```python
from build123d import *

# Parameters (mm, degrees)
SKETCH1_W             = 12
SKETCH1_H             = 12
SKETCH1_R             = 1.65
BOSS_EXTRUDE1_DEPTH   = 7
BOSS_EXTRUDE1_2_DEPTH = 7
BOSS_EXTRUDE1_3_DEPTH = 7
BOSS_EXTRUDE1_4_DEPTH = 7
CUT_EXTRUDE1_START    = -2.25
CUT_EXTRUDE1_DEPTH    = 2.5
SKETCH3_W             = 22
SKETCH3_H             = 12
BOSS_EXTRUDE2_DEPTH   = 7
SKETCH4_W             = 10
SKETCH4_H             = 12
SKETCH4_R             = 1.65
SKETCH4_W_2           = 12
BOSS_EXTRUDE3_DEPTH   = 7
CUT_EXTRUDE2_START    = -2.25
CUT_EXTRUDE2_DEPTH    = 2.5
SKETCH6_W             = 10
SKETCH6_H             = 12
SKETCH6_R             = 1.65
SKETCH6_W_2           = 12
BOSS_EXTRUDE4_DEPTH   = 5


with BuildPart() as part:
    # Sketch1 → Boss-Extrude1 (new body)
    with BuildSketch(Plane(origin=(0, 0, 0), x_dir=(1, 0, 0), z_dir=(0, 1, 0))):
        with Locations((1, 38)):
            Rectangle(SKETCH1_W, SKETCH1_H)
        with Locations((1, 38)):
            Circle(SKETCH1_R, mode=Mode.SUBTRACT)
    extrude(amount=BOSS_EXTRUDE1_DEPTH)


with BuildPart() as body_2:
    # Sketch1 → Boss-Extrude1 2 (new body)
    with BuildSketch(Plane(origin=(0, 0, 0), x_dir=(1, 0, 0), z_dir=(0, 1, 0))):
        with Locations((6, -6)):
            Rectangle(SKETCH1_W, SKETCH1_H)
        with Locations((6, -6)):
            Circle(SKETCH1_R, mode=Mode.SUBTRACT)
    extrude(amount=BOSS_EXTRUDE1_2_DEPTH)


with BuildPart() as body_3:
    # Sketch1 → Boss-Extrude1 3 (new body)
    with BuildSketch(Plane(origin=(0, 0, 0), x_dir=(1, 0, 0), z_dir=(0, 1, 0))):
        with Locations((-10, 18)):
            Rectangle(SKETCH1_W, SKETCH1_H)
        with Locations((-10, 18)):
            Circle(SKETCH1_R, mode=Mode.SUBTRACT)
    extrude(amount=BOSS_EXTRUDE1_3_DEPTH)


with BuildPart() as body_4:
    # Sketch1 → Boss-Extrude1 4 (new body)
    with BuildSketch(Plane(origin=(0, 0, 0), x_dir=(1, 0, 0), z_dir=(0, 1, 0))):
        with Locations((24, 18)):
            Rectangle(SKETCH1_W, SKETCH1_H)
        with Locations((24, 18)):
            Circle(SKETCH1_R, mode=Mode.SUBTRACT)
    extrude(amount=BOSS_EXTRUDE1_4_DEPTH)


with BuildPart() as cut_extrude1_tool:
    # Sketch2 → Cut-Extrude1 (new body)
    with BuildSketch(Plane(origin=(0, 7, 0), x_dir=(1, 0, 0), z_dir=(0, 1, 0)).offset(CUT_EXTRUDE1_START)):
        Polygon((9.233161507, -6), (7.616580754, -3.2), (4.383419246, -3.2), (2.766838493, -6), (4.383419246, -8.8), (7.616580754, -8.8), align=None)
        Polygon((20.766838493, 18), (22.383419246, 15.2), (25.616580754, 15.2), (27.233161507, 18), (25.616580754, 20.8), (22.383419246, 20.8), align=None)
        Polygon((-2.233161507, 38), (-0.616580754, 35.2), (2.616580754, 35.2), (4.233161507, 38), (2.616580754, 40.8), (-0.616580754, 40.8), align=None)
        Polygon((-13.233161507, 18), (-11.616580754, 15.2), (-8.383419246, 15.2), (-6.766838493, 18), (-8.383419246, 20.8), (-11.616580754, 20.8), align=None)
    extrude(amount=-CUT_EXTRUDE1_DEPTH)


with BuildPart() as part_1:
    add(part.part)

    # Cut-Extrude1: cut by cut_extrude1_tool
    add(cut_extrude1_tool.part, mode=Mode.SUBTRACT)



with BuildPart() as body_2_1:
    add(body_2.part)

    # Cut-Extrude1: cut by cut_extrude1_tool
    add(cut_extrude1_tool.part, mode=Mode.SUBTRACT)


with BuildPart() as body_3_1:
    add(body_3.part)

    # Cut-Extrude1: cut by cut_extrude1_tool
    add(cut_extrude1_tool.part, mode=Mode.SUBTRACT)


with BuildPart() as body_4_1:
    add(body_4.part)

    # Cut-Extrude1: cut by cut_extrude1_tool
    add(cut_extrude1_tool.part, mode=Mode.SUBTRACT)


with BuildPart() as part_2:
    add(part_1.part)

    add(body_2_1.part)  # Boss-Extrude2 merges body 2

    add(body_3_1.part)  # Boss-Extrude2 merges body 3

    add(body_4_1.part)  # Boss-Extrude2 merges body 4
    # Sketch3 → Boss-Extrude2 (add)
    with BuildSketch(Plane(origin=(0, 7, 0), x_dir=(1, 0, 0), z_dir=(0, 1, 0))):
        Polygon((-16, 24), (-4, 24), (18, 24), (19, 24), (19, 32), (-16, 32), align=None)
        with Locations((7, 18)):
            Rectangle(SKETCH3_W, SKETCH3_H)
        Polygon((-21, 12), (-21, 0), (0, 0), (12, 0), (30, 0), (30, 12), (18, 12), (-4, 12), align=None)
    extrude(amount=-BOSS_EXTRUDE2_DEPTH)

    # Sketch4 → Boss-Extrude3 (add)
    with BuildSketch(Plane(origin=(0, 7, 0), x_dir=(1, 0, 0), z_dir=(0, 1, 0))):
        with Locations((-11, 38)):
            Rectangle(SKETCH4_W, SKETCH4_H)
        with Locations((-11, 38)):
            Circle(SKETCH4_R, mode=Mode.SUBTRACT)
        with Locations((24, -6)):
            Rectangle(SKETCH4_W_2, SKETCH4_H)
        with Locations((24, -6)):
            Circle(SKETCH4_R, mode=Mode.SUBTRACT)
    extrude(amount=-BOSS_EXTRUDE3_DEPTH)

    # Sketch5 → Cut-Extrude2 (cut)
    with BuildSketch(Plane(origin=(0, 7, 0), x_dir=(1, 0, 0), z_dir=(0, 1, 0)).offset(CUT_EXTRUDE2_START)):
        Polygon((-7.766838493, 38), (-9.383419246, 40.8), (-12.616580754, 40.8), (-14.233161507, 38), (-12.616580754, 35.2), (-9.383419246, 35.2), align=None)
        Polygon((27.233161507, -6), (25.616580754, -3.2), (22.383419246, -3.2), (20.766838493, -6), (22.383419246, -8.8), (25.616580754, -8.8), align=None)
    extrude(amount=-CUT_EXTRUDE2_DEPTH, mode=Mode.SUBTRACT)

    # Sketch6 → Boss-Extrude4 (add)
    with BuildSketch(Plane(origin=(0, 7, 0), x_dir=(1, 0, 0), z_dir=(0, 1, 0))):
        with Locations((-11, 38)):
            Rectangle(SKETCH6_W, SKETCH6_H)
        with Locations((-11, 38)):
            Circle(SKETCH6_R, mode=Mode.SUBTRACT)
        with Locations((24, -6)):
            Rectangle(SKETCH6_W_2, SKETCH6_H)
        with Locations((24, -6)):
            Circle(SKETCH6_R, mode=Mode.SUBTRACT)
    extrude(amount=BOSS_EXTRUDE4_DEPTH)


solid = part_2.part
```
Could you check a few things on this model? Use its own coordinates, in mm. A direction names the side the tool comes from. Give positions to 0.01 mm unless a question says otherwise; leave off trailing zeros. Loops run counter-clockwise (first coordinate to the right, second up) from the corner with the lowest first, then second, coordinate; pieces in that order, holes last. Notation, with made-up numbers: (81, 15) - (137, 15) arc R16 ccw to (137, 46) - close; hole circle Ø11 at (69.25, -2.5). An arc over 180 degrees is marked (long way). Use one line per item in the form item = value.
1. I want a section at B-B (y = 10.5). Please give me the cut outline in (x, z).
Response values:
outline = (-16, -44) - (-6, -44) - (-6, -32) - (-16, -32) - close; (18, 0) - (30, 0) - (30, 12) - (18, 12) - close; hole circle Ø3.3 at (-11, -38); hole circle Ø3.3 at (24, 6)
2. I need wall thicknesses on probe 1 along Z at (x, y) = (24, 6.05); probe 2 along X at (y, z) = (6.35, -18); probe 3 along X at (y, z) = (5.5, 6). Which ranges of each line are inside material? Lowest first, please.
Response values:
probe_1 = -24 to -19.65, -16.35 to 4.35, 7.65 to 12
probe_2 = -16 to -11.65, -8.35 to 22.35, 25.65 to 30
probe_3 = 0 to 4.35, 7.65 to 12, 18 to 22.35, 25.65 to 30
3. Thinking about a two-plate mould opening in Y: for faces 1 (the face through (4.69, 5.86, 7)), 2 (the face through (-12.414, 3.518, -19.42)), 3 (the face through (4, 0, -16)), which applies, released by +Y, released by -Y, zero draft, split by the parting line, or undercut?
Response values:
face_1 = zero draft
face_2 = undercut
face_3 = released by -Y
4. I'm going to push flat-ended pins straight in: pin 1 Ø4.5 at (x, z) = (6, 6) entering from +Y; pin 2 Ø2 at (x, y) = (-6.5, 3) entering from +Z; pin 3 Ø2 at (y, z) = (2.5, -38) entering from -X. Where does each tip first touch, or does it pass through?
Response values:
pin_1 = 7
pin_2 = 0
pin_3 = -16
5. I want a section at A-A (x = 6). Please give me the cut outline in (y, z), and give its area (3 significant figures).
Response values:
outline = (0, -44) - (7, -44) - (7, 4.35) - (4.75, 4.35) - (4.75, 3.2) - (2.25, 3.2) - (2.25, 4.35) - (0, 4.35) - close; (0, 7.65) - (2.25, 7.65) - (2.25, 8.8) - (4.75, 8.8) - (4.75, 7.65) - (7, 7.65) - (7, 12) - (0, 12) - close
area = 363 mm²
6. On a 3-axis mill with a long thin cutter (end or side, diameter ignored), from which of +Z, -Z, +X, -X, +Y, -Y can I reach the whole of each face in a straight line? I mean faces 4 (the face through (3.564, 3.518, 7.38)), 5 (the face through (-16, 5, -31)), 6 (the face through (19, 4, -28)). Say none if no direction works.
Response values:
face_4 = none
face_5 = -Z, -X, +Y, -Y
face_6 = -Z, +X, +Y, -Y
7. I want a section at D-D (x = -10). Give the number of separate pieces and of enclosed holes in the cut face, and give its area (3 significant figures).
Response values:
separate_pieces = 3
enclosed_holes = 0
area = 300 mm²
8. I want a section at C-C (y = 1). Please give me the cut outline in (x, z).
Response values:
outline = (-21, -12) - (-16, -12) - (-16, -44) - (-6, -44) - (-6, -32) - (-5, -32) - (-5, -44) - (7, -44) - (7, -32) - (19, -32) - (19, -24) - (30, -24) - (30, 12) - (18, 12) - (18, 0) - (12, 0) - (12, 12) - (0, 12) - (0, 0) - (-21, 0) - close; hole circle Ø3.3 at (-11, -38); hole circle Ø3.3 at (-10, -18); hole circle Ø3.3 at (1, -38); hole circle Ø3.3 at (6, 6); hole circle Ø3.3 at (24, -18); hole circle Ø3.3 at (24, 6)
